```python
from build123d import *

# Parameters (mm, degrees)
SKETCH1_W           = 38.1
SKETCH1_H           = 88.9
SKETCH1_R           = 2.5
SKETCH1_R_2         = 4
BOSS_EXTRUDE1_DEPTH = 4.7625


with BuildPart() as part:
    # Sketch1 → Boss-Extrude1 (new body)
    with BuildSketch(Plane.XY):
        with Locations((19.05, 44.45)):
            Rectangle(SKETCH1_W, SKETCH1_H)
        with Locations(Location((19.05, 56.45, 0), (0, 0, 180))):
            Circle(SKETCH1_R, mode=Mode.SUBTRACT)
        with Locations(Location((31.05, 44.45, 0), (0, 0, 180))):
            Circle(SKETCH1_R, mode=Mode.SUBTRACT)
        with Locations(Location((19.05, 32.45, 0), (0, 0, 180))):
            Circle(SKETCH1_R, mode=Mode.SUBTRACT)
        with Locations(Location((7.05, 44.45, 0), (0, 0, 180))):
            Circle(SKETCH1_R, mode=Mode.SUBTRACT)
        with Locations(Location((19.05, 15.875, 0), (0, 0, 180))):
            Circle(SKETCH1_R_2, mode=Mode.SUBTRACT)
    extrude(amount=BOSS_EXTRUDE1_DEPTH)


solid = part.part
```
Geometry check sheet. Reference: the model listing, model coordinates, mm. Coordinates: 2 decimals unless noted, no trailing zeros. Write each loop counter-clockwise with the first axis right and the second up, starting at its lowest first coordinate (ties: lowest second). Pieces come first, ordered by that corner, then holes. Notation, with made-up numbers: (24, 42.5) -> (49, 42.5) arc R25 cw to (49, 57.5) -> close; hole circle Ø6 at (23.25, 88.5). An arc over 180 degrees is marked (long way). Use CSV: the item, a comma, the result in double quotes. Start each with the question number.
Item 1: Cross-section at D-D, the plane y = 44.45. Record the cut outline in (x, z), plus the area to 3 significant figures.
Item 2: Cross-section at B-B, the plane y = 56.45. Record the cut outline in (x, z).
Item 3: Depth check by flat-ended pin: pin 1 Ø2 at (x, y) = (22, 26) entering from -Z. Enter the tip coordinate at first touch or a pass-through.
Item 4: Mould release check, pull along Y, two halves, no side actions. Record for faces 1 (the cylindrical face through (19.59, 34.89, 2.35)), 2 (the cylindrical face through (23.046, 15.699, 2.348)), 3 (the flat face through (19, 45, 0)), 4 (the flat face through (19, 0, 2)): released by +Y, released by -Y, zero draft, split by the parting line, or undercut.
Item 5: Cross-section at C-C, the plane x = 31.05. Record the cut outline in (y, z).
Item 6: Thickness scan on line 1 (X direction, y = 44.45, z = 2.6); line 2 (Y direction, x = 19.05, z = 1.3) (3 decimals); line 3 (Y direction, x = 31.05, z = 2.1). Record the ranges inside material, lowest first.
Item 7: Cross-section at A-A, the plane x = 19.05. State how many separate pieces and enclosed holes the cut face has, plus the area to 3 significant figures.
Answers:
1,outline,"(0, 0) -> (4.55, 0) -> (4.55, 4.76) -> (0, 4.76) -> close; (9.55, 0) -> (28.55, 0) -> (28.55, 4.76) -> (9.55, 4.76) -> close; (33.55, 0) -> (38.1, 0) -> (38.1, 4.76) -> (33.55, 4.76) -> close"
1,area,"134 mm^2"
2,outline,"(0, 0) -> (16.55, 0) -> (16.55, 4.76) -> (0, 4.76) -> close; (21.55, 0) -> (38.1, 0) -> (38.1, 4.76) -> (21.55, 4.76) -> close"
3,pin 1,"z = 0"
4,face 1,"undercut"
4,face 2,"undercut"
4,face 3,"zero draft"
4,face 4,"released by -Y"
5,outline,"(0, 0) -> (41.95, 0) -> (41.95, 4.76) -> (0, 4.76) -> close; (46.95, 0) -> (88.9, 0) -> (88.9, 4.76) -> (46.95, 4.76) -> close"
6,line 1,"0 to 4.55, 9.55 to 28.55, 33.55 to 38.1"
6,line 2,"0 to 11.875, 19.875 to 29.95, 34.95 to 53.95, 58.95 to 88.9"
6,line 3,"0 to 41.95, 46.95 to 88.9"
7,separate pieces,"4"
7,enclosed holes,"0"
7,area,"338 mm^2"
